Autodesk Fusion 360 part; units mm, degrees
sketch "Sketch1" plane through (0, 0, 0) normal (0, 1, 0) x (1, 0, 0)
  circle A0 centre (0, 0) radius 17.095
  circle A1 centre (0, 0) radius 32.5
  line L0 (-21.05, 10) -> (-28.55, 10)
  line L1 (-28.55, 10) -> (-28.55, -10)
  line L2 (-28.55, -10) -> (-21.05, -10)
  line L3 (-21.05, -10) -> (-21.05, 10)
  line L4 (-21.05, 0) -> (0, 0)
  line L5 (0, 0) -> (-19.4454, 19.4454)
  circle A2 centre (-19.4454, 19.4454) radius 0.5
  line L6 (-10, -21.05) -> (-10, -28.55)
  line L7 (10, -28.55) -> (10, -21.05)
  line L8 (-10, -28.55) -> (10, -28.55)
  line L9 (10, -21.05) -> (-10, -21.05)
  circle A3 centre (-19.4454, -19.4454) radius 0.5
  line L10 (21.05, -10) -> (28.55, -10)
  line L11 (28.55, 10) -> (21.05, 10)
  line L12 (28.55, -10) -> (28.55, 10)
  line L13 (21.05, 10) -> (21.05, -10)
  circle A4 centre (19.4454, -19.4454) radius 0.5
  line L14 (10, 21.05) -> (10, 28.55)
  line L15 (-10, 28.55) -> (-10, 21.05)
  line L16 (10, 28.55) -> (-10, 28.55)
  line L17 (-10, 21.05) -> (10, 21.05)
  circle A5 centre (19.4454, 19.4454) radius 0.5
  line L18 (17.3241, -8.1317) -> (8.1317, -17.3241)
  line L19 (0, 0) -> (12.7279, -12.7279)
  line L20 (10.253, -19.4454) -> (8.1317, -17.3241)
  line L21 (8.1317, -17.3241) -> (11.3137, -14.1421)
  line L22 (11.3137, -14.1421) -> (13.435, -16.2635)
  line L23 (13.435, -16.2635) -> (10.253, -19.4454)
  line L24 (19.4454, -10.253) -> (17.3241, -8.1317)
  line L25 (17.3241, -8.1317) -> (14.1421, -11.3137)
  line L26 (14.1421, -11.3137) -> (16.2635, -13.435)
  line L27 (16.2635, -13.435) -> (19.4454, -10.253)
  line L28 (11.844, -17.8544) -> (13.6118, -19.6222)
  circle A6 centre (13.6118, -19.6222) radius 0.5
  line L29 (17.8544, -11.844) -> (19.6222, -13.6118)
  circle A7 centre (19.6222, -13.6118) radius 0.5
  circle A8 centre (-13.6118, 19.6222) radius 0.5
  circle A9 centre (-19.6222, 13.6118) radius 0.5
  point P0 (0, -21.05)
  point P1 (21.05, 0)
  point P2 (0, 21.05)
  dimension "d1" = 34.19
  dimension "d2" = 65
  dimension "d4" = 21.05
  dimension "d5" = 20
  dimension "d6" = 7.5
  dimension "d7" = 27.5
  dimension "d8" = 1
  dimension "d9" = 45
  dimension "d11" = 360
  dimension "d13" = 13
  dimension "d14" = 18
  dimension "d15" = 3
  dimension "d16" = 4.5
  dimension "d17" = 3
  dimension "d18" = 4.5
  dimension "d19" = 2.5
  dimension "d20" = 1
  dimension "d21" = 2.5
  dimension "d22" = 1
  dimension "d24" = 360
extrude "Extrude1" add sketch "Sketch1" along normal blind 12.45 contours L0 L1 L2 L3 | L6 L7 L8 L9 | L10 L11 L12 L13 | L14 L15 L16 L17 makes body 1 at (3.3333, 4.15, 21.05) makes body 2 at (21.05, 4.15, -3.3333) makes body 3 at (-21.05, 4.15, 3.3333) makes body 4 at (-3.3333, 4.15, -21.05)
extrude "Extrude2" add sketch "Sketch1" along normal blind 2 contours L18 L24 L25 L26 L27 | L18 L20 L21 L22 L23 | A1 bodies 1 2 3 4
extrude "Extrude3" add 4 faces at (-26.05, 12.45, 3.3333) (-3.3333, 12.45, 23.55) (23.55, 12.45, -3.3333) (3.3333, 12.45, -23.55) along direction (0, 1, 0) blind 1.8 on bodies 1 bodies 1
sketch "Sketch2" plane through (0, 0, 28.55) normal (0, 0, 1) x (1, 0, 0)
  line L0 (-10, 2) -> (10, 2)
  line L1 (10, 2) -> (10, 14.25)
  line L2 (10, 14.25) -> (-10, 14.25)
  line L3 (-10, 14.25) -> (-10, 2)
  circle A0 centre (0, 12.245) radius 1
  dimension "d31" = 2
  dimension "d32" = 12.245
extrude "Extrude4" add 4 faces at (-3.3333, 14.25, 23.55) (23.55, 14.25, -3.3333) (3.3333, 14.25, -23.55) (-26.05, 14.25, 3.3333) along direction (0, 1, 0) blind 3 on bodies 1 bodies 1
sketch "Sketch3" plane through (28.55, 0, 0) normal (1, 0, 0) x (0, 0, -1)
  line L0 (-10, 2) -> (10, 2)
  line L1 (10, 2) -> (10, 17.25)
  line L2 (10, 17.25) -> (-10, 17.25)
  line L3 (-10, 17.25) -> (-10, 2)
  circle A0 centre (0, 12.445) radius 1
  dimension "d35" = 2
  dimension "d36" = 12.445
extrude "Extrude5" cut sketch "Sketch3" against normal blind 60 contours A0 bodies 1
extrude "Extrude6" cut sketch "Sketch2" against normal blind 60 contours A0 bodies 1
sketch "Sketch4" plane through (0, 0, 0) normal (0, 0, 1) x (1, 0, 0)
  line L0 (21.05, 2) -> (21.05, 17.25)
  line L1 (-21.05, 12.445) -> (21.05, 12.445)
  point P0 (-21.05, 12.445)
  point P1 (21.05, 12.445)
sketch "Sketch5" plane through (0, 0, 0) normal (0, 0, 1) x (1, 0, 0)
sketch "Sketch6" plane through (0, 0, 0) normal (0, 0, 1) x (1, 0, 0)
  line L0 (-21.05, 12.445) -> (21.05, 12.445)
  line L1 (-21.05, 12.445) -> (0, 12.445)
  point P0 (-21.05, 12.445)
sphere "SpherePrimitive1" add diameter 38 placed x (1, 0, 0) y (0, 1, 0) z (0, 0, 1) at (0, 12.445, 0) separate body makes body 5
extrude "Extrude7" add sketch "Sketch2" against normal blind 57.1 contours A0 bodies 5 1
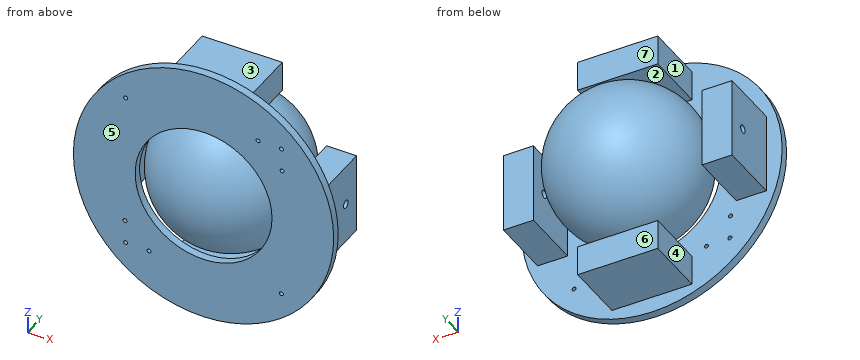
Source: CAD feature listing. Evaluate the final solid. Frame: model axes, mm. Face numbers are marked on the shaded views. A direction names the side the tool comes from. Give positions to 0.01 mm unless a question says otherwise; leave off trailing zeros. Loops run counter-clockwise (first coordinate to the right, second up) from the corner with the lowest first, then second, coordinate; pieces in that order, holes last. Notation, with made-up numbers: (62, 75.5) -> (84, 75.5) arc R16 ccw to (84, 96.5) -> close; hole circle Ø5 at (70.25, 22). An arc over 180 degrees is marked (long way). Put each result on its own line as item: value. Start each with the question number.
1) Draft query along Z for the marked faces 1, 2 and 3. Return one class per face: released by +Z, released by -Z, zero draft, split by the parting line, or undercut.
2) Cut plane B-B (x = 5.5). Return loops of the section in (y, z) (3 decimals), then the cut area to 3 significant figures.
3) Reachability of the marked faces 4, 5, 6 and 7 from +Z, -Z, +X, -X, +Y, -Y: full face, straight path, thin tool, end or side. Return the list, or none.
4) Contact query for flat-ended pins moving along their axis: P1, Ø10, axis at y = 22.5, z = 0, coming from the +X side; P2, Ø17, axis at x = 1.5, y = 13.5, coming from the -Z side; P3, Ø5, axis at x = 3.5, y = 25, coming from the -Z side; P4, Ø12, axis at y = 6, z = -2.5, coming from the -X side. Output: stop coordinate, or through.
5) Material intervals for probe 1 along X at (y, z) = (9, 2); probe 2 along X at (y, z) = (13, -3.5); probe 3 along Y at (x, z) = (25, 0) (3 decimals), sorted ascending.
6) Cut plane A-A (z = 3.5). Return loops of the section in (x, y) (3 decimals), then the cut area to 3 significant figures.
7) Cut plane C-C (y = 6). Return loops of the section in (x, z).
8) Cut plane D-D (x = -26). Return loops of the section in (y, z) (3 decimals), then the cut area to 3 significant figures.
Results are:
1. face 1: zero draft
1. face 2: undercut
1. face 3: released by +Z
2. outline: circle Ø36.373 at (12.445, 0); (0, -32.031) -> (2, -32.031) -> (2, -28.55) -> (17.25, -28.55) -> (17.25, -21.05) -> (2, -21.05) -> (2, -16.186) -> (0, -16.186) -> close; (0, 16.186) -> (2, 16.186) -> (2, 21.05) -> (17.25, 21.05) -> (17.25, 28.55) -> (2, 28.55) -> (2, 32.031) -> (0, 32.031) -> close
2. area: 1,330 mm2
3. face 4: -Z, -X, +Y
3. face 5: -Y
3. face 6: -Z, +X, -X, +Y
3. face 7: +Z, +X, -X, +Y
4. P1: stops at x = 18.32
4. P2: stops at z = -28.55
4. P3: stops at z = -15.81
4. P4: stops at x = -32.5
5. probe 1: x = -28.55 to -21.05, -18.58 to 18.58, 21.05 to 28.55
5. probe 2: x = -28.55 to -21.05, -18.67 to 18.67, 21.05 to 28.55
5. probe 3: y = 0 to 11.445, 13.445 to 17.25
6. outline: (-32.311, 0) -> (-16.733, 0) -> (-16.733, 2) -> (-21.05, 2) -> (-21.05, 17.25) -> (-28.55, 17.25) -> (-28.55, 2) -> (-32.311, 2) -> close; circle Ø37.35 at (0, 12.445); (16.733, 0) -> (32.311, 0) -> (32.311, 2) -> (28.55, 2) -> (28.55, 17.25) -> (21.05, 17.25) -> (21.05, 2) -> (16.733, 2) -> close
6. area: 1,390 mm2
7. outline: (-28.55, -10) -> (-21.05, -10) -> (-21.05, 10) -> (-28.55, 10) -> close; circle Ø35.75 at (0, 0); (-10, -28.55) -> (10, -28.55) -> (10, -21.05) -> (-10, -21.05) -> close; (-10, 21.05) -> (10, 21.05) -> (10, 28.55) -> (-10, 28.55) -> close; (21.05, -10) -> (28.55, -10) -> (28.55, 10) -> (21.05, 10) -> close
8. outline: (0, -19.5) -> (2, -19.5) -> (2, -10) -> (17.25, -10) -> (17.25, 10) -> (2, 10) -> (2, 19.5) -> (0, 19.5) -> close; hole circle Ø2 at (12.445, 0)
8. area: 380 mm2
